Can you work these out from the model? Positions are in its coordinate system, mm. Face numbers are marked on the shaded views. A direction names the side the tool comes from. Give positions to 0.01 mm unless a question says otherwise; leave off trailing zeros. Order: outer loops, then holes, each group sorted by start corner. A loop starts at its lowest first (then second) coordinate and runs counter-clockwise, first axis right, second up. Notation, with made-up numbers: (-39.5, -28) -> (-20.5, -28) arc R25 ccw to (-20.5, 4) -> close; hole circle Ø5 at (18.5, 15.5). An arc over 180 degrees is marked (long way). Answer as CSV lines item,"result".
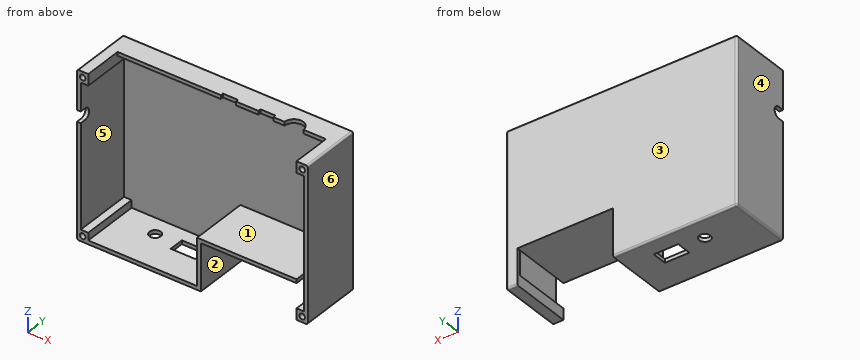
```python
from build123d import *

# Parameters (mm, degrees)
SKETCH2_W                 = 123
SKETCH2_H                 = 88
BOSS_EXTRUDE1_DEPTH       = 2
SKETCH3_W                 = 6
SKETCH3_H                 = 6
CUT_EXTRUDE1_DEPTH        = 2
BOSS_EXTRUDE2_DEPTH       = 33
CUT_EXTRUDE2_DEPTH        = 113.317629961
CUT_EXTRUDE2_DEPTH_BACK   = 2
SKETCH5_W                 = 13
SKETCH5_H                 = 8
SKETCH5_R                 = 3
SKETCH6_W                 = 111
SKETCH6_H                 = 21
CUT_EXTRUDE3_DEPTH        = 2
SKETCH7_W                 = 8
SKETCH7_H                 = 1.5
CUT_EXTRUDE4_DEPTH        = 2
F_3_0MM_DOWEL_HOLE2_D     = 3
F_3_0MM_DOWEL_HOLE2_DEPTH = 15
F_3_0MM_DOWEL_HOLE2_TIP   = 0.901290929
CUT_EXTRUDE10_DEPTH       = 2
FILLET1_R                 = 1


with BuildPart() as part:
    # Sketch2 → Boss-Extrude1 (new body)
    with BuildSketch(Plane(origin=(0, 0, 0), x_dir=(1, 0, 0), z_dir=(0, 1, 0))):
        Rectangle(SKETCH2_W, SKETCH2_H)
    extrude(amount=-BOSS_EXTRUDE1_DEPTH)

    # Sketch3 → Cut-Extrude1 (cut)
    with BuildSketch(Plane(origin=(0, 0, 0), x_dir=(1, 0, 0), z_dir=(0, 1, 0))):
        Polygon((55.5, 38), (55.5, 44), (4.5, 44), (4.5, 19), (55.5, 19), align=None)
        with Locations((58.5, 41)):
            Rectangle(SKETCH3_W, SKETCH3_H)
    extrude(amount=-CUT_EXTRUDE1_DEPTH, mode=Mode.SUBTRACT)

    # Sketch4 → Boss-Extrude2 (add)
    with BuildSketch(Plane(origin=(0, 0, 0), x_dir=(1, 0, 0), z_dir=(0, 1, 0))):
        Polygon((59.5, -38), (55.5, -38), (55.5, -42), (-55.5, -42), (-55.5, -38), (-59.5, -38), (-59.5, 38), (-55.5, 38), (-55.5, 42), (2.5, 42), (2.5, 17), (55.5, 17), (55.5, 19), (4.5, 19), (4.5, 44), (-61.5, 44), (-61.5, -44), (61.5, -44), (61.5, 38), (55.5, 38), (55.5, 32), (59.5, 32), align=None)
    extrude(amount=-BOSS_EXTRUDE2_DEPTH)

    # Sketch5 → Cut-Extrude2 (cut, two sides: drawn at the far end of the back side and taken through both)
    with BuildSketch(Plane(origin=(0, 0, -44), x_dir=(-1, 0, 0), z_dir=(0, 0, -1)).offset(-CUT_EXTRUDE2_DEPTH_BACK)):
        with Locations((17, -13)):
            Rectangle(SKETCH5_W, SKETCH5_H)
        with Locations((35.5, -12)):
            Circle(SKETCH5_R)
    extrude(amount=CUT_EXTRUDE2_DEPTH + CUT_EXTRUDE2_DEPTH_BACK, mode=Mode.SUBTRACT)

    # Sketch6 → Cut-Extrude3 (cut)
    with BuildSketch(Plane.XY.offset(44)):
        with Locations((0, -22.5)):
            Rectangle(SKETCH6_W, SKETCH6_H)
    extrude(amount=-CUT_EXTRUDE3_DEPTH, mode=Mode.SUBTRACT)

    # Sketch7 → Cut-Extrude4 (cut)
    with BuildSketch(Plane.XY.offset(44)):
        with BuildLine():
            Line((33.5, -12), (43.5, -12))
            ThreePointArc((43.5, -12), (38.5, -7), (33.5, -12))
        make_face()
        with Locations((3.5, -11.25)):
            Rectangle(SKETCH7_W, SKETCH7_H)
        with Locations((23.5, -11.25)):
            Rectangle(SKETCH7_W, SKETCH7_H)
    extrude(amount=-CUT_EXTRUDE4_DEPTH, mode=Mode.SUBTRACT)

    # Ø3.0mm Dowel Hole2
    with Locations(Plane(origin=(0, -33, 0), x_dir=(-1, 0, 0), z_dir=(0, -1, 0))):
        with Locations((58.5, -41), (58.5, 41), (-58.5, 35), (-58.5, -41)):
            Hole(F_3_0MM_DOWEL_HOLE2_D / 2, depth=F_3_0MM_DOWEL_HOLE2_DEPTH)
            with Locations((0, 0, -(F_3_0MM_DOWEL_HOLE2_DEPTH + F_3_0MM_DOWEL_HOLE2_TIP / 2))):  # 118° drill point
                Cone(0, F_3_0MM_DOWEL_HOLE2_D / 2, F_3_0MM_DOWEL_HOLE2_TIP, mode=Mode.SUBTRACT)

    # Sketch15 → Cut-Extrude10 (cut)
    with BuildSketch(Plane.ZY.offset(61.5)):
        with BuildLine():
            ThreePointArc((23, -30), (20, -27), (17, -30))
            Line((17, -30), (17, -33))
            Line((17, -33), (23, -33))
            Line((23, -33), (23, -30))
        make_face()
    extrude(amount=-CUT_EXTRUDE10_DEPTH, mode=Mode.SUBTRACT)

    # Fillet1
    fillet1_edges = [part.edges().sort_by_distance(p)[0] for p in [
        (-28.5, 0, -44),
        (61.5, -16.5, -38),
        (58.5, 0, -38),
        (0, 0, 44),
        (-61.5, 0, 0),
        (61.5, 0, 3),
        (61.5, -16.5, 44),
        (-61.5, -16.5, 44),
        (-61.5, -16.5, -44),
    ]]
    fillet(fillet1_edges, radius=FILLET1_R)


solid = part.part
```
Item 1: We'd pull the mould along X, two halves only. Please class the marked faces 4, 5 and 6: released by +X, released by -X, zero draft, split by the parting line, or undercut.
Numbers:
face 4,"released by -X"
face 5,"undercut"
face 6,"released by +X"
Item 2: Imagine slicing it at A-A, the plane y = -25. Give the number of separate pieces and of enclosed holes in the cut face, then the cut area to 3 significant figures.
Numbers:
separate pieces,"2"
enclosed holes,"4"
area,"679 mm²"
Item 3: Please list where these lines run through material, in increasing order: line 1 along Z through (x, y) = (58.5, -26.5); line 2 along X through (y, z) = (-21, -35); line 3 along Z through (x, y) = (-58.5, -21.75).
Numbers:
line 1,"z = -38 to -36.5, -33.5 to -32, 38 to 39.5, 42.5 to 44"
line 2,"x = -61.5 to -59.5, 2.5 to 4.5, 55.5 to 57, 60 to 61.5"
line 3,"z = -44 to -42.5, -39.5 to -38, 38 to 39.5, 42.5 to 44"
Item 4: For pin 1 (2 mm diameter, centred on x = 13, z = 42.5, fed in from -Y); pin 2 (1.6 mm diameter, centred on x = 22, z = 43.5, fed in from -Y); pin 3 (5 mm diameter, centred on x = 4, z = 29.5, fed in from -Y), each with a flat end and sliding along its axis, tell me the tip position at first contact or that it passes through.
Numbers:
pin 1,"stops at y = -12"
pin 2,"stops at y = -10.5"
pin 3,"stops at y = -2"
Item 5: Imagine slicing it at B-B, the plane x = -35.5. Please give me the cut outline in (y, z).
Numbers:
outline,"(-33, -44) -> (-15, -44) -> (-15, -42) -> (-33, -42) -> close; (-12, 42) -> (-2, 42) -> (-2, -42) -> (-9, -42) -> (-9, -44) -> (-1, -44) arc R1 ccw to (0, -43) -> (0, 43) arc R1 ccw to (-1, 44) -> (-12, 44) -> close"
Item 6: Imagine slicing it at D-D, the plane x = 24.5. Please give me the cut outline in (y, z).
Numbers:
outline,"(-33, -19) -> (0, -19) -> (0, 43) arc R1 ccw to (-1, 44) -> (-10.5, 44) -> (-10.5, 42) -> (-2, 42) -> (-2, -17) -> (-33, -17) -> close"
Item 7: For the marked faces 1, 2 and 3, which set-ups out of +Z, -Z, +X, -X, +Y, -Y let a thin tool reach every point of the face, with its end or its side?
Numbers:
face 1,"-Y"
face 2,"-Z, +Y, -Y"
face 3,"+Z, -Z, +X, -X, +Y"
Item 8: Imagine slicing it at C-C, the plane z = 6.5. Please give me the cut outline in (x, y).
Numbers:
outline,"(-61.5, -33) -> (-59.5, -33) -> (-59.5, -2) -> (59.5, -2) -> (59.5, -33) -> (61.5, -33) -> (61.5, -1) arc R1 ccw to (60.5, 0) -> (-60.5, 0) arc R1 ccw to (-61.5, -1) -> close"
